Read the model definition and answer for the solid it produces. Units are mm, in the model's axes. Give positions to 0.01 mm unless a question says otherwise; leave off trailing zeros. Order: outer loops, then holes, each group sorted by start corner. A loop starts at its lowest first (then second) coordinate and runs counter-clockwise, first axis right, second up. Notation, with made-up numbers: M 51,37 L 75,37 A26 cw 75,54 Z; hole C 5,25.5 d8. An arc over 180 degrees is marked long. One line per item, written item: value.
Autodesk Inventor part; units mm, degrees
ref_plane "YZ Plane" through (0, 0, 0) normal (1, 0, 0) x (0, 1, 0)
ref_plane "XZ Plane" through (0, 0, 0) normal (0, 1, 0) x (-1, 0, 0)
ref_plane "XY Plane" through (0, 0, 0) normal (0, 0, 1) x (1, 0, 0)
sketch "Náčrt1" plane through (0, 0, 0) normal (0, 0, 1) x (1, 0, 0)
  line L0 (-10, -10) -> (10, -10)
  line L1 (10, -10) -> (10, 10)
  line L2 (10, 10) -> (-10, 10)
  line L3 (-10, 10) -> (-10, -10)
  line L4 (-10, -10) -> (10, 10) construction
  line L5 (10, -10) -> (-10, 10) construction
  line L6 (-9, -9) -> (9, -9)
  line L7 (9, -9) -> (9, 9)
  line L8 (9, 9) -> (-9, 9)
  line L9 (-9, 9) -> (-9, -9)
  line L10 (-9, -9) -> (9, 9) construction
  line L11 (9, -9) -> (-9, 9) construction
  point P0 (0, 0)
  dimension "d0" = 20
  dimension "d1" = 20
  dimension "d2" = 18
  dimension "d3" = 18
extrude "Vysunutí1" add sketch "Náčrt1" along normal mid plane 355
fillet "Zaoblení1" radius 1 8 edges at (-9, -9, 0) (9, -9, 0) (9, 9, 0) (-9, 9, 0) (10, -10, 0) (10, 10, 0) (-10, 10, 0) (-10, -10, 0)
sketch "Náčrt2" plane through (10, -9, 177.5) normal (1, 0, 0) x (0, 0, -1)
  line L0 (355, 18) -> (355, 0)
  line L1 (0, -1) -> (355, -1)
  point P0 (177.5, 9)
  point P1 (335, 9)
  point P2 (355, 9)
  dimension "d7" = 20
  dimension "d8" = 10
hole "Díra1" at (10, 0, -157.5) direction (-1, 0, 0) diameter 3 end through all
sketch "Náčrt3" plane through (-10, -9, 177.5) normal (-1, 0, 0) x (0, 0, 1)
  line L0 (0, 18) -> (0, 0)
  line L1 (-355, -1) -> (0, -1)
  point P0 (-177.5, 9)
  point P1 (-40, 9)
  point P2 (-140, 9)
  dimension "d16" = 40
  dimension "d17" = 10
  dimension "d18" = 100
  dimension "d19" = 10
hole "Díra2" at (-10, 0, 137.5) at (-10, 0, 37.5) direction (1, 0, 0) diameter 3 end through all
properties part number "Hlavni_pater"
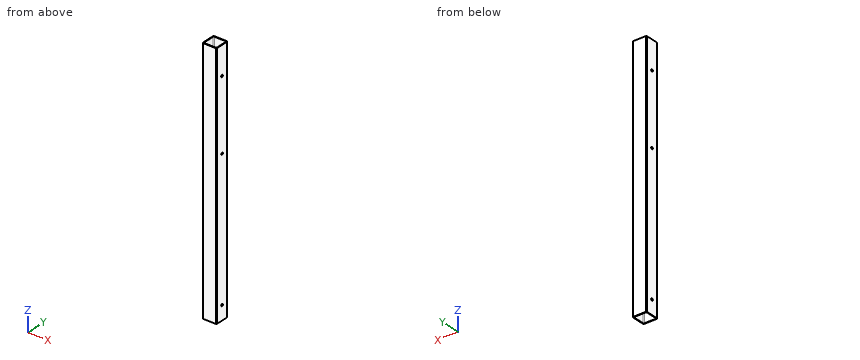
1) Find section C-C, the plane z = 66. Write down the section's boundary in (x, y).
Reported:
outline: M -10,-9 A1 ccw -9,-10 L 9,-10 A1 ccw 10,-9 L 10,9 A1 ccw 9,10 L -9,10 A1 ccw -10,9 Z; hole M -9,-8 A1 ccw -8,-9 L 8,-9 A1 ccw 9,-8 L 9,8 A1 ccw 8,9 L -8,9 A1 ccw -9,8 Z
2) Find section A-A, the plane y = 4.5. Write down the section's boundary in (x, z), plus the area to 3 significant figures.
Reported:
outline: M -10,-177.5 L -9,-177.5 L -9,177.5 L -10,177.5 Z; M 9,-177.5 L 10,-177.5 L 10,177.5 L 9,177.5 Z
area: 710 mm^2
3) This flat-tipped pin is pushed along its axis until it touches: pin 1 Ø3.5 at (y, z) = (0, -157.5) entering from -X. Where does it stop, or does it pass through?
Reported:
pin 1: stops at x = -10
4) Consider probe 1 along Z at (x, y) = (9.6, 0); probe 2 along Y at (x, z) = (-7.5, -115). Determine where each line is inside the solid, lowest interval first.
Reported:
probe 1: z = -177.5 to -159, -156 to 36, 39 to 136, 139 to 177.5
probe 2: y = -10 to -9, 9 to 10
